from build123d import *

# Parameters (mm, degrees)
CYLINDER025_R           = 1.6
CYLINDER025_DEPTH       = 10
CYLINDER025_PITCH_ANGLE = 90
CYLINDER024_R           = 1.6
CYLINDER024_DEPTH       = 10
CYLINDER024_PITCH_ANGLE = 90
BOX040_W                = 3
BOX040_H                = 3
BOX040_DEPTH            = 10
BOX039_W                = 3
BOX039_H                = 3
BOX039_DEPTH            = 10
BOX038_W                = 5
BOX038_H                = 10
BOX038_DEPTH            = 3
ARRAY022_Y_COUNT        = 11
ARRAY022_Y_PITCH        = 20
BOX037_W                = 3
BOX037_H                = 208
BOX037_DEPTH            = 17.6


with BuildPart() as cylinder025:
    # Cylinder025 → Cylinder025 (new body)
    with BuildSketch(Plane.XY):
        Circle(CYLINDER025_R)
    extrude(amount=CYLINDER025_DEPTH)


with BuildPart() as cylinder025_1:
    # Cylinder025 pitch: moved
    add(cylinder025.part.rotate(Axis((0, 0, 0), (0, 1, 0)), CYLINDER025_PITCH_ANGLE))


with BuildPart() as cylinder025_2:
    # Cylinder025 placement: moved
    add(cylinder025_1.part.moved(Location((-5, -25, -5.3))))


with BuildPart() as cylinder024:
    # Cylinder024 → Cylinder024 (new body)
    with BuildSketch(Plane.XY):
        Circle(CYLINDER024_R)
    extrude(amount=CYLINDER024_DEPTH)


with BuildPart() as cylinder024_1:
    # Cylinder024 pitch: moved
    add(cylinder024.part.rotate(Axis((0, 0, 0), (0, 1, 0)), CYLINDER024_PITCH_ANGLE))


with BuildPart() as cylinder024_2:
    # Cylinder024 placement: moved
    add(cylinder024_1.part.moved(Location((-5, -175, -5.3))))


with BuildPart() as cube040:
    # Box040 → Box040 (new body)
    with BuildSketch(Plane(origin=(-4, -204, -3.2), x_dir=(1, 0, 0), z_dir=(0, 0, 1))):
        with Locations((1.5, 1.5)):
            Rectangle(BOX040_W, BOX040_H)
    extrude(amount=BOX040_DEPTH)


with BuildPart() as cube039:
    # Box039 → Box039 (new body)
    with BuildSketch(Plane(origin=(-4, 1, -3.2), x_dir=(1, 0, 0), z_dir=(0, 0, 1))):
        with Locations((1.5, 1.5)):
            Rectangle(BOX039_W, BOX039_H)
    extrude(amount=BOX039_DEPTH)


with BuildPart() as array022:
    # Box038 → Box038 (new body)
    with BuildSketch(Plane(origin=(-1, -1, 7), x_dir=(1, 0, 0), z_dir=(0, 0, 1))):
        with Locations((2.5, 5)):
            Rectangle(BOX038_W, BOX038_H)
    extrude(amount=BOX038_DEPTH)

    # Array022 Y: Array022 ×11


with BuildPart() as array022_1:
    add(array022.part)
    with Locations(*[(0, i * ARRAY022_Y_PITCH, 0) for i in range(1, ARRAY022_Y_COUNT)]):
        add(array022.part)


with BuildPart() as sidepanel01:
    # Box037 → Box037 (new body)
    with BuildSketch(Plane.XY.offset(-7.6)):
        with Locations((1.5, 104)):
            Rectangle(BOX037_W, BOX037_H)
    extrude(amount=BOX037_DEPTH)

    # Cut035: cut Array022
    add(array022_1.part, mode=Mode.SUBTRACT)


with BuildPart() as sidepanel01_1:
    # Cut035 placement: moved
    add(sidepanel01.part.moved(Location((-4, -204, -1.2))))

    # Cut036: cut Cube039
    add(cube039.part, mode=Mode.SUBTRACT)

    # Cut037: cut Cube040
    add(cube040.part, mode=Mode.SUBTRACT)

    # Cut050: cut Cylinder024
    add(cylinder024_2.part, mode=Mode.SUBTRACT)

    # Cut051: cut Cylinder025
    add(cylinder025_2.part, mode=Mode.SUBTRACT)


solid = sidepanel01_1.part
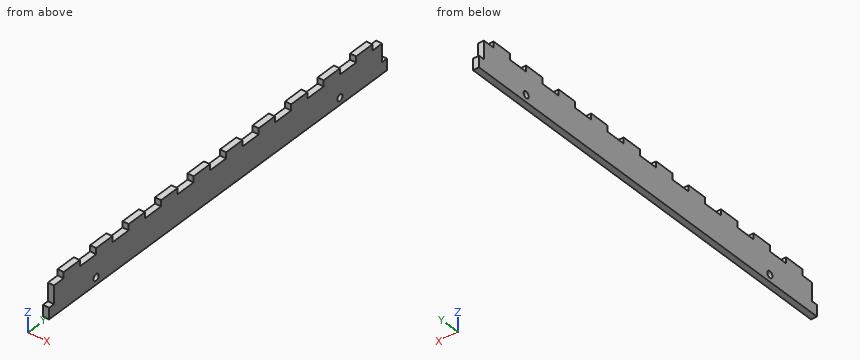
Geometry: final body of the model. Coordinates: model frame, mm. Round coordinates to 2 decimals unless told otherwise and drop trailing zeros. Loops run counter-clockwise (first coordinate to the right, second up) from the corner with the lowest first, then second, coordinate; pieces in that order, holes last. Notation, with made-up numbers: (85.5, 37.25) - (113.5, 37.25) arc R17 ccw to (113.5, 58.25) - close; hole circle Ø7 at (57.5, -34.5). An arc over 180 degrees is marked (long way). Write each question's results on one line, items separated by ' | '. Start each with the question number.
1) Cut plane A-A on z = 1. Return loops of the section in (x, y), then the cut area to 3 significant figures.
2) First-contact query: P1, Ø0.9, axis at x = -2.5, z = 6.5, coming from the -Y side; P2, Ø1.5, axis at x = -2, y = -144, coming from the +Z side; P3, Ø0.9, axis at x = -3, z = 2, coming from the -Y side. Flat tips, straight axial feed; report the tip coordinate or a pass-through.
3) Cut plane B-B on x = -2.45. Count the separate pieces of the cut face and the enclosed holes in it, then the cut area to 3 significant figures.
4) Cut plane C-C on y = -98.5. Return loops of the section in (x, z).
5) Line query: probe 1 along Y at (x, z) = (-2.3, -5.3); probe 2 along Y at (x, z) = (-3.65, 5); probe 3 along Z at (x, y) = (-1.5, -42). Output: solid intervals per line, ascending. Write a range as [from, to].
Verdict:
1) outline: (-4, -201) - (-1, -201) - (-1, 1) - (-4, 1) - close | area: 606 mm2
2) P1: stops at y = -195 | P2: stops at z = 5.8 | P3: stops at y = -201
3) separate pieces: 1 | enclosed holes: 2 | area: 3,270 mm2
4) outline: (-4, -8.8) - (-1, -8.8) - (-1, 5.8) - (-4, 5.8) - close
5) probe 1: y = [-204, -176.6], [-173.4, -26.6], [-23.4, 4] | probe 2: y = [-201, 1] | probe 3: z = [-8.8, 5.8]
